from build123d import *

# Parameters (mm, degrees)
SKETCH1_W           = 98.806
SKETCH1_H           = 33.02
BOSS_EXTRUDE1_DEPTH = 0.4572
CUT_EXTRUDE1_DEPTH  = 1.4572


with BuildPart() as part:
    # Sketch1 → Boss-Extrude1 (new body)
    with BuildSketch(Plane(origin=(0, 0, 0), x_dir=(1, 0, 0), z_dir=(0, 1, 0))):
        Rectangle(SKETCH1_W, SKETCH1_H)
    extrude(amount=BOSS_EXTRUDE1_DEPTH)

    # Sketch2 → Cut-Extrude1 (cut, through all)
    with BuildSketch(Plane(origin=(0, 0.4572, 0), x_dir=(1, 0, 0), z_dir=(0, 1, 0))):
        with BuildLine():
            Line((-12.7, 3.81), (12.7, 3.81))
            ThreePointArc((12.7, 3.81), (16.51, 0), (12.7, -3.81))
            Line((12.7, -3.81), (-12.7, -3.81))
            ThreePointArc((-12.7, -3.81), (-16.51, 0), (-12.7, 3.81))
        make_face()
    extrude(amount=-CUT_EXTRUDE1_DEPTH, mode=Mode.SUBTRACT)


solid = part.part
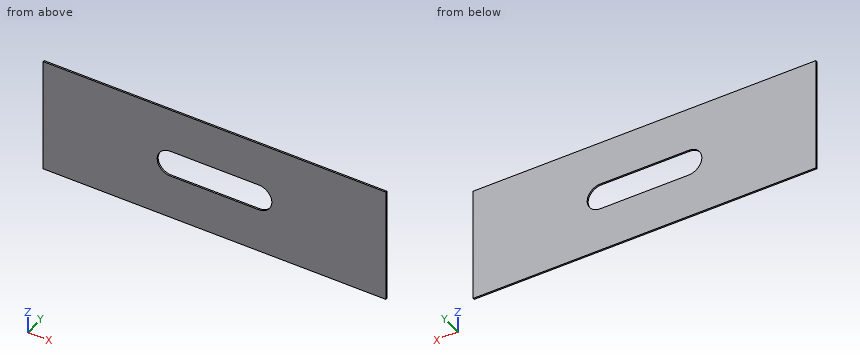
Work out the finished part from the listing and answer in its coordinate system (mm). Give positions to 0.01 mm unless a question says otherwise; leave off trailing zeros. Write each loop counter-clockwise with the first axis right and the second up, starting at its lowest first coordinate (ties: lowest second). Pieces come first, ordered by that corner, then holes.
Q1. The part is cut by section B-B on x = -10.5. Give the vertices of the cut face in (y, z), and give its area (3 significant figures).
Answer:
outline: (0, -16.51) - (0.46, -16.51) - (0.46, -3.81) - (0, -3.81) - close; (0, 3.81) - (0.46, 3.81) - (0.46, 16.51) - (0, 16.51) - close
area: 11.6 mm2
Q2. Straight lines are drawn through the part: L1, parallel to Z at x = -3.5, y = 0.25; L2, parallel to X at y = 0.4, z = -0.5. For each, find the intervals that lie inside material, in ascending order.
Answer:
L1: z = -16.51 to -3.81, 3.81 to 16.51
L2: x = -49.4 to -16.48, 16.48 to 49.4
Q3. The part is cut by section A-A on z = 0. Give the vertices of the cut face in (x, y).
Answer:
outline: (-49.4, 0) - (-16.51, 0) - (-16.51, 0.46) - (-49.4, 0.46) - close; (16.51, 0) - (49.4, 0) - (49.4, 0.46) - (16.51, 0.46) - close
Q4. The part is cut by section C-C on y = 0.1. Give the vertices of the cut face in (x, z), and give its area (3 significant figures).
Answer:
outline: (-49.4, -16.51) - (49.4, -16.51) - (49.4, 16.51) - (-49.4, 16.51) - close; hole (-12.7, -3.81) - (12.7, -3.81) arc R3.81 ccw to (12.7, 3.81) - (-12.7, 3.81) arc R3.81 ccw to start
area: 3,020 mm2
